Autodesk Inventor part; units mm, degrees
ref_plane "YZ Plane" through (0, 0, 0) normal (1, 0, 0) x (0, 1, 0)
ref_plane "XZ Plane" through (0, 0, 0) normal (0, 1, 0) x (-1, 0, 0)
ref_plane "XY Plane" through (0, 0, 0) normal (0, 0, 1) x (1, 0, 0)
sketch "Skizze1" plane through (0, 0, 0) normal (0, 1, 0) x (-1, 0, 0)
  line L0 (0, 0) -> (155, 0)
  line L1 (155, 0) -> (155, -85)
  line L2 (155, -85) -> (0, -85)
  line L3 (0, -85) -> (0, 0)
  dimension "d0" = 155
  dimension "d1" = 85
extrude "Extrusion1" add sketch "Skizze1" along normal blind 22
sketch "Skizze2" plane through (0, 22, 0) normal (0, 1, 0) x (1, 0, 0)
  line L0 (-1.5, 1.5) -> (-153.5, 1.5)
  line L1 (-153.5, 1.5) -> (-153.5, 83.5)
  line L2 (-153.5, 83.5) -> (-1.5, 83.5)
  line L3 (-1.5, 83.5) -> (-1.5, 1.5)
  line L4 (-155, 0) -> (0, 0)
  line L5 (0, 85) -> (-155, 85)
  line L6 (0, 0) -> (0, 85)
  line L7 (-155, 85) -> (-155, 0)
  dimension "d4" = 1.5
  dimension "d5" = 1.5
  dimension "d6" = 1.5
  dimension "d7" = 1.5
extrude "Extrusion2" cut sketch "Skizze2" against normal blind 20.5 contours L0 L1 L2 L3
sketch "Skizze3" plane through (-155, 0, 0) normal (0, 0, 1) x (1, 0, 0)
  line L0 (27.2, 17.8) -> (39.2, 17.8)
  line L1 (40.2, 16.8) -> (40.2, 11.8)
  line L2 (39.2, 10.8) -> (27.2, 10.8)
  line L3 (26.2, 11.8) -> (26.2, 16.8)
  arc A0 (26.2, 11.8) -> (27.2, 10.8) centre (27.2, 11.8) ccw
  arc A1 (27.2, 17.8) -> (26.2, 16.8) centre (27.2, 16.8) ccw
  arc A2 (40.2, 16.8) -> (39.2, 17.8) centre (39.2, 16.8) ccw
  arc A3 (39.2, 10.8) -> (40.2, 11.8) centre (39.2, 11.8) ccw
  line L4 (153.5, 1.5) -> (1.5, 1.5)
  line L5 (1.5, 22) -> (1.5, 1.5)
  point P0 (155, 0)
  dimension "d10" = 1
  dimension "d71" = 14
  dimension "d72" = 7
  dimension "d73" = 9.3
  dimension "d74" = 24.7
extrude "Extrusion3" cut sketch "Skizze3" against normal blind 3
sketch "Skizze4" plane through (0, 1.5, 0) normal (0, 1, 0) x (1, 0, 0)
  circle A0 centre (-80.95, 23.5) radius 2.75
  circle A1 centre (-80.95, 61.5) radius 2.75
  circle A2 centre (-23.95, 23.5) radius 2.75
  circle A3 centre (-23.95, 61.5) radius 2.75
  circle A4 centre (-80.95, 23.5) radius 1.2
  circle A5 centre (-80.95, 61.5) radius 1.2
  circle A6 centre (-23.95, 23.5) radius 1.2
  circle A7 centre (-23.95, 61.5) radius 1.2
  line L0 (-1.5, 83.5) -> (-1.5, 1.5)
  line L1 (-1.5, 1.5) -> (-153.5, 1.5)
  line L2 (-153.5, 83.5) -> (-1.5, 83.5)
  point P0 (0, 0)
  dimension "d13" = 5.5
  dimension "d14" = 5.5
  dimension "d15" = 5.5
  dimension "d16" = 5.5
  dimension "d17" = 38
  dimension "d18" = 38
  dimension "d19" = 57
  dimension "d40" = 2.4
  dimension "d41" = 2.4
  dimension "d42" = 2.4
  dimension "d43" = 2.4
  dimension "d44" = 22.45
  dimension "d45" = 22
  dimension "d47" = 22
  dimension "d51" = 22.45
  dimension "d53" = 57
  dimension "d54" = 22
  dimension "d55" = 22
extrude "Extrusion4" add sketch "Skizze4" along normal blind 5.5
sketch "Skizze5" plane through (-155, 0, -85) normal (-1, 0, 0) x (0, 0, 1)
  line L0 (15.5, 8.6) -> (24.5, 8.6)
  line L1 (24.5, 8.6) -> (24.5, 13.6)
  line L2 (24.5, 13.6) -> (15.5, 13.6)
  line L3 (15.5, 13.6) -> (15.5, 8.6)
  line L4 (1.5, 22) -> (1.5, 1.5)
  line L5 (83.5, 1.5) -> (1.5, 1.5)
  point P0 (85, 0)
  dimension "d59" = 14
  dimension "d60" = 9
  dimension "d61" = 5
  dimension "d62" = 7.1
extrude "Extrusion5" cut sketch "Skizze5" against normal blind 3
fillet "Rundung1" radius 1 4 edges at (0, 11, 0) (0, 11, -85) (-155, 11, 0) (-155, 11, -85)
fillet "Rundung2" radius 1 8 edges at (-0.2929, 0, -0.2929) (0, 0, -42.5) (-0.2929, 0, -84.7071) (-77.5, 0, -85) (-154.7071, 0, -84.7071) (-155, 0, -42.5) (-154.7071, 0, -0.2929) (-77.5, 0, 0)
sketch "Skizze6" plane through (0, 0, 0) normal (0, -1, 0) x (1, 0, 0)
  circle A0 centre (-140, -70) radius 6.5
  circle A1 centre (-140, -15) radius 6.5
  circle A2 centre (-15, -70) radius 6.5
  circle A3 centre (-15, -15) radius 6.5
  line L0 (-1, 0) -> (-154, 0)
  line L1 (-154, -85) -> (-1, -85)
  line L2 (-155, -1) -> (-155, -84)
  line L3 (0, -84) -> (0, -1)
  point P0 (0, 0)
  dimension "d26" = 13
  dimension "d27" = 13
  dimension "d28" = 13
  dimension "d29" = 13
  dimension "d63" = 15
  dimension "d64" = 15
  dimension "d65" = 15
  dimension "d66" = 15
  dimension "d67" = 15
  dimension "d68" = 15
  dimension "d69" = 15
  dimension "d70" = 15
extrude "Extrusion6" cut sketch "Skizze6" against normal blind 0.2
sketch "Skizze7" plane through (-1, 22, -85) normal (0, 0, -1) x (-1, 0, 0)
  circle A0 centre (128.2, -10) radius 1.5
  circle A1 centre (117.6, -10) radius 1.5
  line L0 (152.5, -20.5) -> (0.5, -20.5)
  line L1 (152.5, 0) -> (152.5, -20.5)
  point P0 (-1, -22)
  dimension "d35" = 3
  dimension "d36" = 3
  dimension "d37" = 10.6
  dimension "d56" = 10.5
  dimension "d57" = 10.5
  dimension "d58" = 24.3
extrude "Extrusion7" cut sketch "Skizze7" against normal blind 3
properties part number "Datapad_Case"
Design review of the part built by this model. Coordinates are the model's own, in mm. A direction names the side the tool comes from. Give positions to 0.01 mm unless a question says otherwise; leave off trailing zeros. Order: outer loops, then holes, each group sorted by start corner. A loop starts at its lowest first (then second) coordinate and runs counter-clockwise, first axis right, second up. Notation, with made-up numbers: M 0.5,83.25 L 33.5,83.25 A19 ccw 33.5,101.25 Z; hole C 59,4.5 d8. An arc over 180 degrees is marked long. One line per question, with ' | ' between items. Start each with the question number.
Q1. For pin 1 Ø2 at (x, z) = (-108, -35.5) entering from -Y; pin 2 Ø1.9 at (x, z) = (-80.95, -23.5) entering from +Y; pin 3 Ø6 at (x, z) = (-22, -27.5) entering from +Y; pin 4 Ø8 at (x, z) = (-15, -70) entering from -Y, all flat-tipped, find the tip position at first contact; note any pin that passes through.
Q2. Machinability: for faces 1 (the face through (-140, 0.2, -15)), 2 (the face through (-79.47, 4.21, -59.18)), 3 (the face through (-76, 0, -42)), which of the approach directions +Z, -Z, +X, -X, +Y, -Y give a long, thin tool a straight path to every point of the face, cutting with its end or side? Answer none if there is none.
Q3. The part is to be moulded in two halves that separate along Z. For faces 4 (the face through (-155, 11, -42)), 5 (the face through (-76, 11, 0)), 6 (the face through (-79, 12, -83.5)), 7 (the face through (-24.308, 4.212, -20.773)), say which applies: +Z half, -Z half, draft (parallel to the pull), parting line (faces both ways), or undercut.
Q4. We need section D-D (x = -15). Write out the cut boundary in (y, z), plus the area to 3 significant figures.
Q5. We need section C-C (y = 19.5). Write out the cut boundary in (x, z), plus the area to 3 significant figures.
Q6. We need section B-B (x = -108). Write out the cut boundary in (y, z).
Q7. For L1, parallel to X at y = 4, z = -61.5; L2, parallel to X at y = 10, z = -51.5; L3, parallel to Z at x = -41, y = 9, list the stretches that pass through material, from the lowest coordinate up. Write a range as [from, to].
Q8. We need section A-A (z = -41). Write out the cut boundary in (x, y), plus the area to 3 significant figures.
Returned:
1) pin 1: y = 0 | pin 2: y = 1.5 | pin 3: y = 7 | pin 4: y = 0.2
2) face 1: -Y | face 2: +Y | face 3: +Z, -Z, +X, -X, -Y
3) face 4: draft | face 5: +Z half | face 6: undercut | face 7: undercut
4) outline: M 0,-84 A1 ccw 1,-85 L 22,-85 L 22,-83.5 L 1.5,-83.5 L 1.5,-1.5 L 22,-1.5 L 22,0 L 1,0 A1 ccw 0,-1 L 0,-8.5 L 0.2,-8.5 L 0.2,-21.5 L 0,-21.5 L 0,-63.5 L 0.2,-63.5 L 0.2,-76.5 L 0,-76.5 Z | area: 183 mm2
5) outline: M -155,-84 A1 ccw -154,-85 L -1,-85 A1 ccw 0,-84 L 0,-1 A1 ccw -1,0 L -154,0 A1 ccw -155,-1 Z; hole M -153.5,-83.5 L -1.5,-83.5 L -1.5,-1.5 L -153.5,-1.5 Z | area: 710 mm2
6) outline: M 0,-84 A1 ccw 1,-85 L 22,-85 L 22,-83.5 L 1.5,-83.5 L 1.5,-1.5 L 22,-1.5 L 22,0 L 1,0 A1 ccw 0,-1 Z
7) L1: [-155, -153.5], [-83.7, -82.15], [-79.75, -78.2], [-26.7, -25.15], [-22.75, -21.2], [-1.5, 0] | L2: [-155, -153.5], [-1.5, 0] | L3: [-85, -83.5], [-1.5, 0]
8) outline: M -155,1 A1 ccw -154,0 L -1,0 A1 ccw 0,1 L 0,22 L -1.5,22 L -1.5,1.5 L -153.5,1.5 L -153.5,22 L -155,22 Z | area: 294 mm2
